For this review, take the finished solid that the model builds, in its own axes (mm). A direction names the side the tool comes from. Round coordinates to 2 decimals unless told otherwise and drop trailing zeros. Use one line per item in the form item = value. Start each with the question number.
Item 1: Add section A-A (z = 0). Count the separate pieces of the cut face and the enclosed holes in it, and give its area (3 significant figures).
Item 2: For P1, Ø4, axis at x = 12.5, z = 28, coming from the +Y side; P2, Ø3, axis at x = -37.5, y = 0, coming from the -Z side; P3, Ø3.5, axis at y = 3, z = 2.5, coming from the +X side, all flat-tipped, find the tip position at first contact; note any pin that passes through.
Item 3: For line 1 (Z direction, x = 0, y = -1.5); line 2 (Z direction, x = 0, y = 1); line 3 (Y direction, x = -6, z = 38.5), list the stretches that pass through material, from the lowest coordinate up. Write a range as [from, to].
Item 4: For faces 1 (the cylindrical face through (-33.727, -1.687, 25.861)), 2 (the flat face through (-0.083, 5.846, 24.53)), 3 (the flat face through (-36, 3, -6)), list the 3-axis set-ups (+Z, -Z, +X, -X, +Y, -Y) from which the entire face can be reached by the end or side of a thin tool; tool diameter is ignored.
Item 5: Draft analysis for pull direction Y (two halves, no side actions). For faces 4 (the flat face through (-36, -1.9, 0)), 5 (the flat face through (9, 2.2, 34)), 6 (the cylindrical face through (34.97, 1.08, -1.45)), 7 (the cylindrical face through (-7.684, 1.037, -1.009)), state which applies: released by +Y, released by -Y, zero draft, split by the parting line, or undercut.
Autodesk Inventor part; units mm, degrees
ref_plane "YZ Plane" through (0, 0, 0) normal (1, 0, 0) x (0, 1, 0)
ref_plane "XZ Plane" through (0, 0, 0) normal (0, 1, 0) x (-1, 0, 0)
ref_plane "XY Plane" through (0, 0, 0) normal (0, 0, 1) x (1, 0, 0)
sketch "スケッチ1" plane through (0, 0, 0) normal (0, 1, 0) x (-1, 0, 0)
  circle A0 centre (0, 0) radius 35
  dimension "d0" = 70
extrude "押し出し1" add sketch "スケッチ1" along normal blind 2.2
sketch "スケッチ2" plane through (0, 2.2, 0) normal (0, 1, 0) x (1, 0, 0)
  circle A0 centre (0, 0) radius 42.5
  line L0 (-3.2969, -22.0057) -> (4.4145, -22.0057) construction
  line L1 (4.4145, -22.0057) -> (4.4145, -25.1797) construction
  line L2 (4.4145, -25.1797) -> (-3.2969, -25.1797) construction
  line L3 (-3.2969, -25.1797) -> (-3.2969, -22.0057) construction
  dimension "d3" = 85
extrude "押し出し2" add sketch "スケッチ2" along normal blind 3.4
chamfer "面取り1" distance 0.75 angle 45 1 edges at (-42.5, 2.2, 0)
chamfer "面取り2" distance 0.75 angle 45 1 edges at (-42.5, 5.6, 0)
sketch "スケッチ3" plane through (0, 0, 0) normal (0, -1, 0) x (1, 0, 0)
  circle A0 centre (0, 0) radius 42.5
  dimension "d12" = 85
extrude "押し出し3" add sketch "スケッチ3" along normal blind 3.4
chamfer "面取り3" distance 0.75 angle 45 1 edges at (-42.5, 0, 0)
chamfer "面取り4" distance 0.75 angle 45 1 edges at (-42.5, -3.4, 0)
sketch "スケッチ6" plane through (0, 5.6, 0) normal (0, 1, 0) x (1, 0, 0)
  circle A0 centre (0, 0) radius 7.65
  line L0 (0, 7.65) -> (46.8799, 7.65)
  circle A1 centre (0, 0) radius 47.5
  line L1 (0, -7.65) -> (46.8799, -7.65)
  dimension "d39" = 15.3
extrude "押し出し5" [suppressed]
chamfer "面取り7" [suppressed]
chamfer "面取り8" [suppressed]
chamfer "面取り9" [suppressed]
sketch "スケッチ7" plane through (0, 5.6, 0) normal (0, 1, 0) x (1, 0, 0)
  line L0 (-9.3358, -20.9354) -> (21.308, -20.9354) construction
  line L1 (21.308, -20.9354) -> (21.308, -27.5341) construction
  line L2 (21.308, -27.5341) -> (-9.3358, -27.5341) construction
  line L3 (-9.3358, -27.5341) -> (-9.3358, -20.9354) construction
  spline S0 degree 2 poles (-5.7914, -21.6571) (-5.2131, -21.667) (-4.2541, -22.0526) (-3.9377, -22.3739) knots 0 0 0 1 2 2 2
  spline S1 degree 2 poles (-3.9377, -22.3739) (-3.646, -22.6754) (-3.3247, -23.5207) (-3.3247, -24.0645) knots 0 0 0 1 2 2 2
  spline S2 degree 2 poles (-3.3247, -24.0645) (-3.3247, -24.633) (-3.6708, -25.5079) (-3.9772, -25.8045) knots 0 0 0 1 2 2 2
  spline S3 degree 2 poles (-3.9772, -25.8045) (-4.3084, -26.1308) (-5.2773, -26.4916) (-5.7914, -26.5015) knots 0 0 0 1 2 2 2
  line L4 (-5.7914, -26.5015) -> (-5.7914, -27.2084)
  line L5 (-5.7914, -27.2084) -> (-6.6021, -27.2084)
  line L6 (-6.6021, -27.2084) -> (-6.6021, -26.5015)
  spline S4 degree 2 poles (-6.6021, -26.5015) (-7.1162, -26.4867) (-8.0802, -26.1506) (-8.4213, -25.8144) knots 0 0 0 1 2 2 2
  spline S5 degree 2 poles (-8.4213, -25.8144) (-8.7277, -25.5129) (-9.0688, -24.628) (-9.0688, -24.0645) knots 0 0 0 1 2 2 2
  spline S6 degree 2 poles (-9.0688, -24.0645) (-9.0688, -23.5306) (-8.7426, -22.6853) (-8.446, -22.3788) knots 0 0 0 1 2 2 2
  spline S7 degree 2 poles (-8.446, -22.3788) (-8.1296, -22.0526) (-7.1805, -21.672) (-6.6021, -21.6571) knots 0 0 0 1 2 2 2
  line L7 (-6.6021, -21.6571) -> (-6.6021, -21.0096)
  line L8 (-6.6021, -21.0096) -> (-5.7914, -21.0096)
  line L9 (-5.7914, -21.0096) -> (-5.7914, -21.6571)
  spline S8 degree 2 poles (-5.7914, -25.8886) (-5.4207, -25.8787) (-4.8473, -25.6562) (-4.6594, -25.4684) knots 0 0 0 1 2 2 2
  spline S9 degree 2 poles (-4.6594, -25.4684) (-4.4073, -25.2212) (-4.17, -24.5143) (-4.17, -24.0299) knots 0 0 0 1 2 2 2
  spline S10 degree 2 poles (-4.17, -24.0299) (-4.17, -23.6245) (-4.3974, -22.9572) (-4.6248, -22.7249) knots 0 0 0 1 2 2 2
  spline S11 degree 2 poles (-4.6248, -22.7249) (-4.8374, -22.5024) (-5.4009, -22.2899) (-5.7914, -22.28) knots 0 0 0 1 2 2 2
  line L10 (-5.7914, -22.28) -> (-5.7914, -25.8886)
  spline S12 degree 2 poles (-6.6021, -22.28) (-6.9926, -22.2849) (-7.5562, -22.5074) (-7.7687, -22.7249) knots 0 0 0 1 2 2 2
  spline S13 degree 2 poles (-7.7687, -22.7249) (-7.9961, -22.9523) (-8.2235, -23.6344) (-8.2235, -24.0299) knots 0 0 0 1 2 2 2
  spline S14 degree 2 poles (-8.2235, -24.0299) (-8.2235, -24.5143) (-7.9862, -25.2262) (-7.7341, -25.4684) knots 0 0 0 1 2 2 2
  spline S15 degree 2 poles (-7.7341, -25.4684) (-7.5463, -25.6463) (-6.9729, -25.8836) (-6.6021, -25.8886) knots 0 0 0 1 2 2 2
  line L11 (-6.6021, -25.8886) -> (-6.6021, -22.28)
  line L12 (1.2181, -21.9735) -> (-1.4216, -27.159)
  line L13 (-1.4216, -27.159) -> (-2.2916, -27.159)
  line L14 (-2.2916, -27.159) -> (0.4964, -21.7758)
  line L15 (0.4964, -21.7758) -> (-2.6525, -21.7758)
  line L16 (-2.6525, -21.7758) -> (-2.6525, -21.059)
  line L17 (-2.6525, -21.059) -> (1.2181, -21.059)
  line L18 (1.2181, -21.059) -> (1.2181, -21.9735)
  spline S16 degree 2 poles (5.761, -24.109) (5.761, -25.7502) (4.8069, -27.2875) (3.8134, -27.2875) knots 0 0 0 1 2 2 2
  spline S17 degree 2 poles (3.8134, -27.2875) (2.8049, -27.2875) (1.8608, -25.7205) (1.8608, -24.1139) knots 0 0 0 1 2 2 2
  spline S18 degree 2 poles (1.8608, -24.1139) (1.8608, -22.4629) (2.8148, -20.9354) (3.8134, -20.9354) knots 0 0 0 1 2 2 2
  spline S19 degree 2 poles (3.8134, -20.9354) (4.8168, -20.9354) (5.761, -22.5173) (5.761, -24.109) knots 0 0 0 1 2 2 2
  spline S20 degree 2 poles (4.713, -25.9677) (4.8317, -25.6661) (4.9305, -24.7368) (4.9305, -24.109) knots 0 0 0 1 2 2 2
  spline S21 degree 2 poles (4.9305, -24.109) (4.9305, -23.4812) (4.8317, -22.5568) (4.7081, -22.2454) knots 0 0 0 1 2 2 2
  spline S22 degree 2 poles (4.7081, -22.2454) (4.5845, -21.9339) (4.1544, -21.6126) (3.8134, -21.6126) knots 0 0 0 1 2 2 2
  spline S23 degree 2 poles (3.8134, -21.6126) (3.4723, -21.6126) (3.0323, -21.9339) (2.9038, -22.2553) knots 0 0 0 1 2 2 2
  spline S24 degree 2 poles (2.9038, -22.2553) (2.7802, -22.5667) (2.6912, -23.5158) (2.6912, -24.1139) knots 0 0 0 1 2 2 2
  spline S25 degree 2 poles (2.6912, -24.1139) (2.6912, -24.7566) (2.7703, -25.6167) (2.8988, -25.9528) knots 0 0 0 1 2 2 2
  spline S26 degree 2 poles (2.8988, -25.9528) (3.0175, -26.2692) (3.4574, -26.6103) (3.8134, -26.6103) knots 0 0 0 1 2 2 2
  spline S27 degree 2 poles (3.8134, -26.6103) (4.1495, -26.6103) (4.5894, -26.289) (4.713, -25.9677) knots 0 0 0 1 2 2 2
  point P0 (0, 0)
extrude "押し出し6" add sketch "スケッチ7" along normal blind 0.5
sketch "スケッチ8" plane through (0, 5.6, 0) normal (0, 1, 0) x (1, 0, 0)
  line L0 (-33, 6) -> (-39, 6)
  line L1 (-39, 6) -> (-39, -6)
  line L2 (-39, -6) -> (-33, -6)
  line L3 (-33, -6) -> (-33, 6)
  arc A0 (-35, 0) -> (-35, 0) centre (0, 0) ccw
  point P0 (-36, -6)
  point P1 (-36, 6)
  dimension "d53" = 12
  dimension "d54" = 6
  dimension "d55" = 33
extrude "押し出し7" cut sketch "スケッチ8" against normal blind 7.5 contours L3 L2 A0 L0 | A0 L2 L1 L0 picked at (-33.6474, -0.6696)
sketch "スケッチ9" plane through (0, 5.6, 0) normal (0, 1, 0) x (1, 0, 0)
  point P0 (0, 0)
  point P1 (0, 0)
hole "穴2" at (0, 5.6, 0) direction (0, -1, 0) diameter 15.5 end through all
sketch "スケッチ10" plane through (0, 5.6, 0) normal (0, 1, 0) x (1, 0, 0)
  circle A0 centre (0, 0) radius 12.5 construction
  point P0 (0, -12.5)
  point P1 (12.5, 0)
  point P2 (0, 12.5)
  point P3 (-12.5, 0)
  dimension "d67" = 25
  dimension "d81" = 360
hole "穴3" at (0, 5.6, 12.5) at (-12.5, 5.6, 0) at (0, 5.6, -12.5) at (12.5, 5.6, 0) direction (0, -1, 0) diameter 3.2 end through all
properties part number "pully_shoulder2_70"
Calculated:
q1.separate_pieces = 5
q1.enclosed_holes = 0
q1.area = 496 mm^2
q2.P1 = 5.6
q2.P2 = -22.27
q2.P3 = 42.49
q3.line_1 = [-42.5, -14.1], [-10.9, -7.75], [7.75, 10.9], [14.1, 42.5]
q3.line_2 = [-35, -14.1], [-10.9, -7.75], [7.75, 10.9], [14.1, 35]
q3.line_3 = [-3.4, 0], [2.2, 5.6]
q4.face_1 = +Y, -Y
q4.face_2 = +Z, +Y
q4.face_3 = +Y
q5.face_4 = released by +Y
q5.face_5 = undercut
q5.face_6 = undercut
q5.face_7 = zero draft
